Source: CAD feature listing. Evaluate the final solid. Frame: model axes, mm. A direction names the side the tool comes from. Give positions to 0.01 mm unless a question says otherwise; leave off trailing zeros. Order: outer loops, then holes, each group sorted by start corner. A loop starts at its lowest first (then second) coordinate and runs counter-clockwise, first axis right, second up.
1) Section B-B, the plane x = 4.5. Return loops of the section in (y, z).
2) Section A-A, the plane z = -8.5. Return loops of the section in (x, y).
3) Section C-C, the plane y = 32. Give the number of separate pieces and of enclosed holes in the cut face, plus the area to 3 significant figures.
4) Access query for faces 5 (the face through (-56.142, 19.227, 63.653)), 6 (the face through (-20, 19, 72.29)). Directions: +Z, -Z, +X, -X, +Y, -Y. A direction counts if a zero-diameter tool reaches every point of the face in a straight line with its end or side. Return the directions, or none.
5) Material intervals for line 1 (X direction, y = 5, z = -24.5); line 2 (Z direction, x = 19, y = 12.5); line 3 (Z direction, x = -56.5, y = 18), sorted ascending.
6) Draft query along Z for faces 1 (the face through (40.646, 19.227, 65.047)), 2 (the face through (-8, 19, -48.03)), 3 (the face through (48.284, 19, -1)), 4 (the face through (-7, 19, -53.11)). Return one class per face: released by +Z, released by -Z, zero draft, split by the parting line, or undercut.
```python
from build123d import *

# Parameters (mm, degrees)
SKETCH1_R           = 1
BOSS_EXTRUDE3_DEPTH = 39
FILLET1_R           = 2.54


with BuildPart() as part:
    # Sketch1 → Boss-Extrude3 (new body)
    with BuildSketch(Plane(origin=(0, 0, 0), x_dir=(1, 0, 0), z_dir=(0, 1, 0))):
        with BuildLine():
            Line((48.284490735, 53.109977813), (-64.735509285, 53.109977813))
            Line((-64.735509285, 53.109977813), (-64.735509285, -72.290076187))
            Line((-64.735509285, -72.290076187), (22.884490735, -72.290076187))
            ThreePointArc((22.884490735, -72.290076187), (40.845002977, -64.850588429), (48.284490735, -46.890076187))
            Line((48.284490735, -46.890076187), (48.284490735, 53.109977813))
        make_face()
        with Locations((-59.655509285, 48.029977813)):
            Circle(SKETCH1_R, mode=Mode.SUBTRACT)
        with Locations((43.204490735, 48.029977813)):
            Circle(SKETCH1_R, mode=Mode.SUBTRACT)
        with Locations((-59.655509285, -67.210076187)):
            Circle(SKETCH1_R, mode=Mode.SUBTRACT)
        with Locations((37.880892571, -60.748479124)):
            Circle(SKETCH1_R, mode=Mode.SUBTRACT)
        with BuildLine():
            Line((38.204490735, 48.029977813), (-54.655509285, 48.029977813))
            ThreePointArc((-54.655509285, 48.029977813), (-56.119975379, 44.494443907), (-59.655509285, 43.029977813))
            Line((-59.655509285, 43.029977813), (-59.655509285, -62.210076187))
            ThreePointArc((-59.655509285, -62.210076187), (-56.119975379, -63.674542281), (-54.655509285, -67.210076187))
            Line((-54.655509285, -67.210076187), (22.884490735, -67.210076187))
            ThreePointArc((22.884490735, -67.210076187), (28.683169352, -66.365130135), (33.999606769, -63.900561058))
            ThreePointArc((33.999606769, -63.900561058), (34.208776178, -57.355020535), (40.717513048, -56.63100608))
            ThreePointArc((40.717513048, -56.63100608), (42.572931676, -51.916774238), (43.204490735, -46.890076187))
            Line((43.204490735, -46.890076187), (43.204490735, 43.029977813))
            ThreePointArc((43.204490735, 43.029977813), (39.668956829, 44.494443907), (38.204490735, 48.029977813))
        make_face(mode=Mode.SUBTRACT)
    extrude(amount=BOSS_EXTRUDE3_DEPTH)

    # Fillet1
    fillet1_edges = [part.edges().sort_by_distance(p)[0] for p in [
        (33.999606769, 19.5, 63.900561058),
        (40.717513048, 19.5, 56.63100608),
        (43.204490735, 19.5, -43.029977813),
        (38.204490735, 19.5, -48.029977813),
        (-54.655509285, 19.5, -48.029977813),
        (-59.655509285, 19.5, -43.029977813),
        (-59.655509285, 19.5, 62.210076187),
        (-54.655509285, 19.5, 67.210076187),
        (-64.735509285, 19.5, 72.290076187),
        (-64.735509285, 19.5, -53.109977813),
        (48.284490735, 19.5, -53.109977813),
    ]]
    fillet(fillet1_edges, radius=FILLET1_R)


solid = part.part
```
From the geometry:
1. outline: (0, -53.11) - (39, -53.11) - (39, -48.03) - (0, -48.03) - close; (0, 67.21) - (39, 67.21) - (39, 72.29) - (0, 72.29) - close
2. outline: (-64.74, 0) - (-59.66, 0) - (-59.66, 39) - (-64.74, 39) - close; (43.2, 0) - (48.28, 0) - (48.28, 39) - (43.2, 39) - close
3. separate pieces: 1
3. enclosed holes: 5
3. area: 2,350 mm2
4. face 5: +Y, -Y
4. face 6: +Z, +X, -X, +Y, -Y
5. line 1: x = -64.74 to -59.66, 43.2 to 48.28
5. line 2: z = -53.11 to -48.03, 67.21 to 72.29
5. line 3: z = -53.11 to -44.15, 63.33 to 72.29
6. face 1: released by +Z
6. face 2: undercut
6. face 3: zero draft
6. face 4: released by -Z
